Geometry check sheet. Reference: the model listing, model coordinates, mm. A direction names the side the tool comes from. Give positions to 0.01 mm unless a question says otherwise; leave off trailing zeros. Write each loop counter-clockwise with the first axis right and the second up, starting at its lowest first coordinate (ties: lowest second). Pieces come first, ordered by that corner, then holes.
(1) Cross-section at B-B (x = 155). Record the boundary of the cut face in (y, z), and give its area (3 significant figures).
(2) Depth check by flat-ended pin: P1, Ø12, axis at x = 150, z = 14, coming from the +Y side; P2, Ø6, axis at y = 4, z = 43.5, coming from the -X side; P3, Ø1.5, axis at x = 77, y = 0.5, coming from the +Z side. Enter the tip coordinate at first touch or a pass-through.
(3) Tool access check on faces 5 (the flat face through (203.2, 0, 44)), 6 (the cylindrical face through (-7.67, 0.34, 25.04)). Record the directions out of +Z, -Z, +X, -X, +Y, -Y that give a thin tool (end or side, any length) a straight path to the whole face; none if there is none.
(4) Cross-section at D-D (z = 26.5). Record the boundary of the cut face in (x, y), and give its area (3 significant figures).
(5) Cross-section at A-A (y = 0). Record the boundary of the cut face in (x, z).
(6) Thickness scan on line 1 along Z through (x, y) = (164, -4); line 2 along X through (y, z) = (0.5, 48.5); line 3 along Z through (x, y) = (184.5, -5.5). Record the ranges inside material, lowest first.
(7) Cross-section at C-C (z = 46.5). Record the boundary of the cut face in (x, y), and give its area (3 significant figures).
(8) Mould release check, pull along Z, two halves, no side actions. Record for faces 1 (the cylindrical face through (102.46, -1.35, 5.59)), 2 (the flat face through (0, 0, 50.8)), 3 (the cylindrical face through (102.23, -1.414, 37.045)), 4 (the flat face through (203.2, 0, 12)): +Z half, -Z half, draft (parallel to the pull), parting line (faces both ways), or undercut.
```python
from build123d import *

# Parameters (mm, degrees)
F0_R     = 7.675775
F1_DEPTH = 50.8
F2_R     = 6.521337
F3_DEPTH = 203.2
F4_R     = 6.217419
F5_DEPTH = 203.2


with BuildPart() as f1:
    # F0 (on Top) → F1 (new body)
    with BuildSketch(Plane.XY):
        Circle(F0_R)
    extrude(amount=F1_DEPTH)

    # F2 (on Right) → F3 (join)
    with BuildSketch(Plane.YZ):
        with Locations((0, 43.410912)):
            Circle(F2_R)
    extrude(amount=F3_DEPTH)

    # F4 (on Right) → F5 (join)
    with BuildSketch(Plane.YZ):
        with Locations((0, 11.660909)):
            Circle(F4_R)
    extrude(amount=F5_DEPTH)


solid = f1.part
```
Reply:
1. outline: circle Ø13.04 at (0, 43.41); circle Ø12.43 at (0, 11.66)
1. area: 255 mm2
2. P1: stops at y = 6.22
2. P2: stops at x = -7.61
2. P3: stops at z = 49.93
3. face 5: +Z, -Z, +X, +Y, -Y
3. face 6: none
4. outline: circle Ø15.35 at (0, 0)
4. area: 185 mm2
5. outline: (-7.68, 0) - (7.68, 0) - (7.68, 5.44) - (203.2, 5.44) - (203.2, 17.88) - (7.68, 17.88) - (7.68, 36.89) - (203.2, 36.89) - (203.2, 49.93) - (7.68, 49.93) - (7.68, 50.8) - (-7.68, 50.8) - close
6. line 1: z = 6.9 to 16.42, 38.26 to 48.56
6. line 2: x = -7.66 to 203.2
6. line 3: z = 8.76 to 14.56, 39.91 to 46.91
7. outline: (5.09, -5.74) - (203.2, -5.74) - (203.2, 5.74) - (5.09, 5.74) arc R7.68 ccw (long way) to start
7. area: 2,440 mm2
8. face 1: undercut
8. face 2: +Z half
8. face 3: undercut
8. face 4: draft
